Can you work these out from the model? Positions are in its coordinate system, mm. Face numbers are marked on the shaded views. A direction names the side the tool comes from. Round coordinates to 2 decimals unless told otherwise and drop trailing zeros. Loops run counter-clockwise (first coordinate to the right, second up) from the corner with the lowest first, then second, coordinate; pieces in that order, holes last.
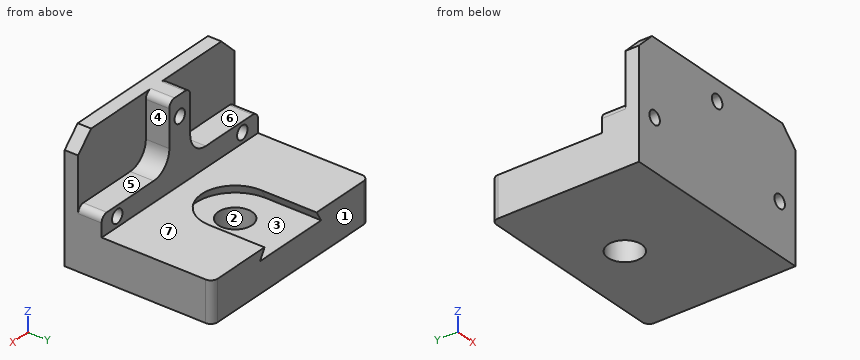
Autodesk Inventor part; units mm, degrees
ref_plane "YZ Plane" through (0, 0, 0) normal (1, 0, 0) x (0, 1, 0)
ref_plane "XZ Plane" through (0, 0, 0) normal (0, 1, 0) x (-1, 0, 0)
ref_plane "XY Plane" through (0, 0, 0) normal (0, 0, 1) x (1, 0, 0)
sketch "Sketch1" plane through (0, 0, 0) normal (0, 1, 0) x (-1, 0, 0)
  line L0 (60, -74) -> (-60, -74)
  line L1 (-60, -74) -> (-60, 0)
  line L2 (-60, 0) -> (60, 0)
  line L3 (60, 0) -> (60, -74)
  point P0 (0, 0)
  point P1 (0, 0)
  dimension "d0" = 120
  dimension "d1" = 74
extrude "Extrusion1" add sketch "Sketch1" along normal blind 8
chamfer "Chamfer1" distance 10 angle 45 2 edges at (60, 4, 0) (-60, 4, 0)
sketch "Sketch2" plane through (0, 8, 0) normal (0, 1, 0) x (1, 0, 0)
  line L0 (-50, 0) -> (-60, 10)
  line L1 (-50, 0) -> (50, 0)
  line L2 (60, 10) -> (60, 74)
  line L3 (60, 74) -> (-60, 74)
  line L4 (-60, 74) -> (-60, 10)
  line L5 (-60, 38) -> (-20, 38)
  line L6 (-8, 26) -> (-8, 0)
  line L7 (-8, 0) -> (-50, 0)
  line L8 (-60, 10) -> (-60, 38)
  arc A0 (-8, 26) -> (-20, 38) centre (-20, 26) ccw
  line L9 (0, 88.8) -> (0, -14.8) construction
  line L10 (50, 0) -> (60, 10)
  line L11 (60, 38) -> (20, 38)
  line L12 (8, 26) -> (8, 0)
  line L13 (8, 0) -> (50, 0)
  line L14 (60, 10) -> (60, 38)
  arc A1 (20, 38) -> (8, 26) centre (20, 26) ccw
  point P0 (0, 0)
  point P1 (8, 0)
  dimension "d7" = 12
  dimension "d8" = 38
  dimension "d9" = 16
extrude "Extrusion2" add sketch "Sketch2" along normal blind 14 contours L6 A0 L5 L4 L3 L2 L11 A1 L12 L1
sketch "Sketch3" plane through (0, 22, 0) normal (0, 1, 0) x (1, 0, 0)
  line L0 (-60, 74) -> (-60, 38)
  line L1 (60, 38) -> (60, 74)
  line L2 (60, 74) -> (-60, 74)
  line L3 (-60, 74) -> (-60, 10)
  line L4 (-60, 74) -> (60, 74)
  line L5 (60, 74) -> (60, 50)
  line L6 (60, 50) -> (-60, 50)
  line L7 (-60, 50) -> (-60, 74)
  point P0 (0, 0)
  point P1 (-60, 50)
  dimension "d12" = 24
extrude "Extrusion3" add sketch "Sketch3" along normal blind 66
fillet "Fillet1" radius 4 6 edges at (60, 88, -62) (-60, 88, -62) (-60, 15, -38) (-8, 15, 0) (8, 15, 0) (60, 15, -38)
sketch "Sketch4" plane through (0, 88, 0) normal (0, 1, 0) x (1, 0, 0)
  line L0 (-56, 50) -> (56, 50)
  line L1 (-20, 50) -> (-23.4641, 56)
  line L2 (-23.4641, 56) -> (23.4641, 56)
  line L3 (60, 50) -> (-60, 50)
  line L4 (23.4641, 56) -> (20, 50)
  line L5 (0, 88.8) -> (0, -14.8) construction
  point P0 (0, 0)
  dimension "d16" = 60
  dimension "d17" = 40
  dimension "d18" = 6
extrude "Extrusion4" cut sketch "Sketch4" against normal blind 33
sketch "Sketch5" plane through (0, 55, 0) normal (0, 1, 0) x (1, 0, 0)
  line L0 (-20, 50) -> (-23.4641, 56)
  line L1 (20, 50) -> (-20, 50)
  line L2 (-23.4641, 56) -> (23.4641, 56)
  line L3 (-20, 50) -> (0, 50)
  line L4 (60, 50) -> (-60, 50)
  line L5 (0, 50) -> (0, 56)
  line L6 (0, 56) -> (-23.4641, 56)
  point P0 (0, 0)
revolve "Revolution1" cut sketch "Sketch5" angle 360 about axis through (0, 55, -50) along (0, 0, -1)
sketch "Sketch6" plane through (-23.4641, 88, -56) normal (0, 0, 1) x (1, 0, 0)
  arc A0 (3.4641, -33) -> (43.4641, -33) centre (23.4641, -33) ccw
  point P0 (23.4641, -88)
hole "Hole1" at (0, 55, -56) direction (0, 0, -1) diameter 20 end through all
sketch "Sketch7" plane through (0, 22, 0) normal (0, 1, 0) x (1, 0, 0)
  line L0 (-4, 0) -> (4, 0)
  line L1 (-50, 0) -> (-4, 0)
  line L2 (0, 88.9657) -> (0, -15.7941) construction
  point P0 (0, 0)
  point P1 (-48, 44)
  point P2 (48, 44)
  point P3 (0, 12)
  point P4 (0, 0)
  dimension "d29" = 44
  dimension "d30" = 96
  dimension "d31" = 12
hole "Hole2" at (-48, 22, -44) at (48, 22, -44) at (0, 22, -12) direction (0, -1, 0) diameter 8 end through all
properties part number "Part019. Corner block" material "Steel, Carbon"
(1) For the marked faces 5, 6 and 7, which set-ups out of +Z, -Z, +X, -X, +Y, -Y let a thin tool reach every point of the face, with its end or its side?
Worked answers:
face 5: +Z, +X, +Y
face 6: +Z, -X, +Y
face 7: +Z, +X, -X, +Y
(2) If we section it at A-A, the plane x = 48: List the corners of the cut face in (y, z) for me, then the cut area to 3 significant figures.
Worked answers:
outline: (0, -74) - (88, -74) - (88, -50) - (22, -50) - (22, -48) - (0, -48) - close; (0, -40) - (22, -40) - (22, -38) - (8, -38) - (8, 0) - (0, 0) - close
area: 2,500 mm2
(3) If we section it at C-C, the plane z = -12: List the corners of the cut face in (x, y) for me, then the cut area to 3 significant figures.
Worked answers:
outline: (-60, 0) - (-4, 0) - (-4, 22) - (-8, 22) - (-8, 8) - (-60, 8) - close; (4, 0) - (60, 0) - (60, 8) - (8, 8) - (8, 22) - (4, 22) - close
area: 1,010 mm2
(4) If I drill on line 1 (X direction, y = 5.5, z = -44); line 2 (Z direction, x = 48, y = 16.5); line 3 (X direction, y = 55, z = -68), over which ranges is the centre line in solid material (lowest first)?
Worked answers:
line 1: x = -60 to -52, -44 to 44, 52 to 60
line 2: z = -74 to -48, -40 to -38
line 3: x = -60 to -10, 10 to 60
(5) If we section it at B-B, the plane z = -44: List the corners of the cut face in (x, y) for me, then the cut area to 3 significant figures.
Worked answers:
outline: (-60, 0) - (-52, 0) - (-52, 22) - (-60, 22) - close; (-44, 0) - (44, 0) - (44, 22) - (-44, 22) - close; (52, 0) - (60, 0) - (60, 22) - (52, 22) - close
area: 2,290 mm2
(6) Will these pins go through, and if not, where does the flat tip stop? P1, Ø6.5, axis at x = -48, z = -44, coming from the -Y side; P2, Ø15.5, axis at x = 37.5, y = 18.5, coming from the +Z side; P3, Ø3, axis at x = 13, y = 65, coming from the +Z side; P4, Ø15.5, axis at y = 17.5, z = -14, coming from the +X side.
Worked answers:
P1: passes through
P2: stops at z = -38
P3: stops at z = -56
P4: stops at x = 8
(7) If we section it at D-D, the plane y = 18.5: List the corners of the cut face in (x, z) for me.
Worked answers:
outline: (-60, -74) - (60, -74) - (60, -42) arc R4 ccw to (56, -38) - (20, -38) arc R12 cw to (8, -26) - (8, -4) arc R4 ccw to (4, 0) - (-4, 0) arc R4 ccw to (-8, -4) - (-8, -26) arc R12 cw to (-20, -38) - (-56, -38) arc R4 ccw to (-60, -42) - close; hole circle Ø8 at (-48, -44); hole circle Ø8 at (0, -12); hole circle Ø8 at (48, -44)
(8) If we mould it in two halves opening along X, with no side actions, what happens to the marked faces 1, 2, 3 and 4? For each: released by +X, released by -X, zero draft, split by the parting line, or undercut.
Worked answers:
face 1: zero draft
face 2: undercut
face 3: undercut
face 4: released by +X
